Verification items for the finished model (mm, model axes). Give positions to 0.01 mm unless a question says otherwise; leave off trailing zeros. Loops run counter-clockwise (first coordinate to the right, second up) from the corner with the lowest first, then second, coordinate; pieces in that order, holes last. Notation, with made-up numbers: (8.5, 8) - (25.5, 8) arc R23 ccw to (25.5, 18) - close; hole circle Ø8 at (83, 85). An arc over 180 degrees is marked (long way). Put each result on its own line as item: value. Start each with the question number.
```python
from build123d import *

# Parameters (mm, degrees)
SKETCH_1_W        = 50
SKETCH_1_H        = 200
EXTRUDE_1_DEPTH   = 2
CHAMFER_1_SIZE    = 2
HOLE_WIZARD_M81_D = 9


with BuildPart() as part:
    # Эскиз1 → Бобышка-Вытянуть1 (new body)
    with BuildSketch(Plane.XY):
        Rectangle(SKETCH_1_W, SKETCH_1_H)
    extrude(amount=EXTRUDE_1_DEPTH)

    # Фаска1
    chamfer_1_edges = [part.edges().sort_by_distance(p)[0] for p in [
        (25, -100, 1),
        (-25, -100, 1),
        (-25, 100, 1),
        (25, 100, 1),
    ]]
    chamfer(chamfer_1_edges, length=CHAMFER_1_SIZE)

    # Отверстие с зазором M81 (through all)
    with Locations(Plane.XY.offset(2)):
        with Locations((0, 75), (0, 25), (0, -25), (0, -75)):
            Hole(HOLE_WIZARD_M81_D / 2)


solid = part.part
```
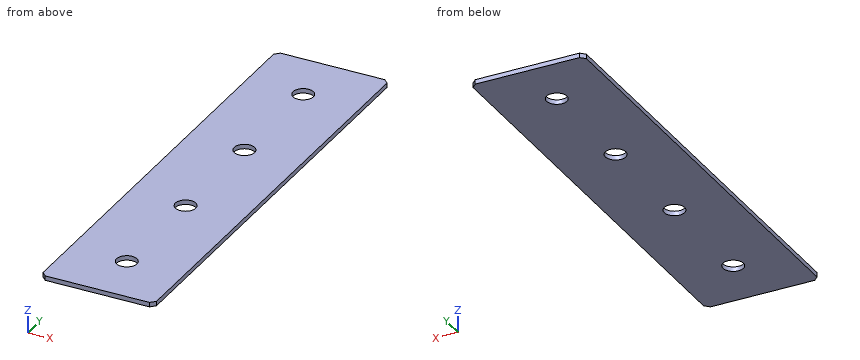
1) Section check B-B, the plane z = 1.6. Enter the section's corners in (x, y), plus the area to 3 significant figures.
2) Section check C-C, the plane x = -1. Enter the section's corners in (y, z), plus the area to 3 significant figures.
3) Depth check by flat-ended pin: P1, Ø5.5, axis at x = 0, y = -75, coming from the +Z side. Enter the tip coordinate at first touch or a pass-through.
4) Section check A-A, the plane y = -25. Enter the section's corners in (x, z).
5) Scan lines: line 1 along Y through (x, z) = (0, 0.55); line 2 along X through (y, z) = (-22.5, 0.5). Record each from-to range of solid material in increasing order. Write a range as from..to.
Results are:
1. outline: (-25, -98) - (-23, -100) - (23, -100) - (25, -98) - (25, 98) - (23, 100) - (-23, 100) - (-25, 98) - close; hole circle Ø9 at (0, -75); hole circle Ø9 at (0, -25); hole circle Ø9 at (0, 25); hole circle Ø9 at (0, 75)
1. area: 9,740 mm2
2. outline: (-100, 0) - (-79.39, 0) - (-79.39, 2) - (-100, 2) - close; (-70.61, 0) - (-29.39, 0) - (-29.39, 2) - (-70.61, 2) - close; (-20.61, 0) - (20.61, 0) - (20.61, 2) - (-20.61, 2) - close; (29.39, 0) - (70.61, 0) - (70.61, 2) - (29.39, 2) - close; (79.39, 0) - (100, 0) - (100, 2) - (79.39, 2) - close
2. area: 330 mm2
3. P1: passes through
4. outline: (-25, 0) - (-4.5, 0) - (-4.5, 2) - (-25, 2) - close; (4.5, 0) - (25, 0) - (25, 2) - (4.5, 2) - close
5. line 1: y = -100..-79.5, -70.5..-29.5, -20.5..20.5, 29.5..70.5, 79.5..100
5. line 2: x = -25..-3.74, 3.74..25
